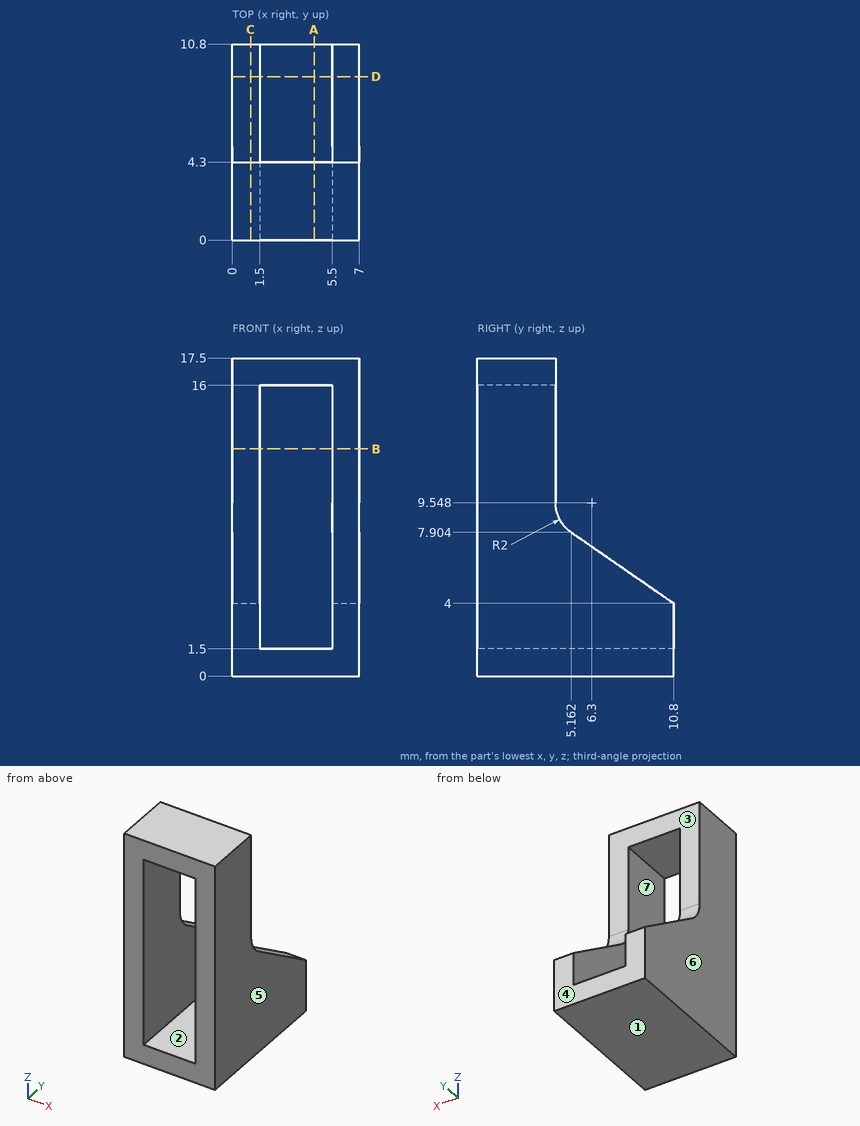
Can you work these out from the drawing? Everything is in mm from the part's minimum corner. A direction names the side the tool comes from. Round coordinates to 2 decimals unless told otherwise and drop trailing zeros. Loops run counter-clockwise (first coordinate to the right, second up) from the corner with the lowest first, then second, coordinate; pieces in that order, holes last. Notation, with made-up numbers: (46, -37.5) - (83, -37.5) arc R30 cw to (83, -10.5) - close; hole circle Ø1 at (53.25, 27). An arc over 180 degrees is marked (long way). One line per question, with ' | ' between items. Start each with the question number.
Q1. I want a section at A-A (x = 4.5). Write out the boundary of the cut face in (y, z).
Q2. We'd pull the mould along X, two halves only. Please class the marked faces 4, 5, 6 and 7: +X half, -X half, draft (parallel to the pull), parting line (faces both ways), or undercut.
Q3. Will these pins go through, and if not, where does the flat tip stop? pin 1 (1 mm diameter, centred on x = 4.5, y = 4, fed in from -Z); pin 2 (1.5 mm diameter, centred on x = 2, y = 7.5, fed in from +Z); pin 3 (3.5 mm diameter, centred on x = 2, z = 12.5, fed in from +Y).
Q4. For the marked faces 1, 2 and 3, which set-ups out of +Z, -Z, +X, -X, +Y, -Y let a thin tool reach every point of the face, with its end or its side?
Q5. I want a section at D-D (y = 9). Write out the boundary of the cut face in (x, z).
Q6. I want a section at B-B (z = 12.5). Write out the boundary of the cut face in (x, y).
Q7. I want a section at C-C (x = 1). Write out the boundary of the cut face in (y, z).
Q8. Please list where these lines run through material, in increasing order: line 1 (X direction, y = 10.25, z = 4.25); line 2 (Z direction, x = 4, y = 3); line 3 (Y direction, x = 5.75, z = 13.5). Write a range as [from, to].
Response values:
1) outline: (0, 0) - (10.8, 0) - (10.8, 1.5) - (0, 1.5) - close; (0, 16) - (4.3, 16) - (4.3, 17.5) - (0, 17.5) - close
2) face 4: draft | face 5: +X half | face 6: -X half | face 7: undercut
3) pin 1: stops at z = 0 | pin 2: stops at z = 6.67 | pin 3: stops at y = 4.3
4) face 1: -Z, +X, -X, +Y, -Y | face 2: +Y, -Y | face 3: +Z, +X, -X, +Y
5) outline: (0, 0) - (7, 0) - (7, 5.25) - (5.5, 5.25) - (5.5, 1.5) - (1.5, 1.5) - (1.5, 5.25) - (0, 5.25) - close
6) outline: (0, 0) - (1.5, 0) - (1.5, 4.3) - (0, 4.3) - close; (5.5, 0) - (7, 0) - (7, 4.3) - (5.5, 4.3) - close
7) outline: (0, 0) - (10.8, 0) - (10.8, 4) - (5.16, 7.9) arc R2 cw to (4.3, 9.55) - (4.3, 17.5) - (0, 17.5) - close
8) line 1: x = [0, 1.5], [5.5, 7] | line 2: z = [0, 1.5], [16, 17.5] | line 3: y = [0, 4.3]
